Can you work these out from the model? Positions are in its coordinate system, mm. Give positions to 0.01 mm unless a question says otherwise; leave off trailing zeros. Order: outer loops, then holes, each group sorted by start corner. A loop starts at its lowest first (then second) coordinate and runs counter-clockwise, first axis right, second up. Notation, with made-up numbers: (27.25, -11.5) - (54.25, -11.5) arc R6 cw to (54.25, -5.5) - close; hole circle Ø4 at (-2.5, -18). An arc over 180 degrees is marked (long way). Return JSON: item names as keys, results as strings.
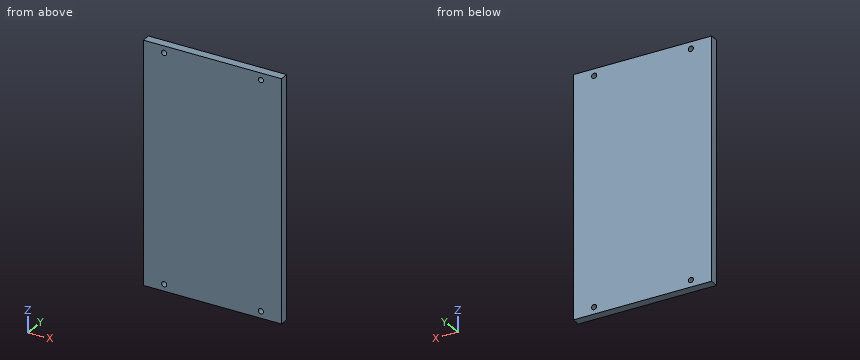
```python
from build123d import *

# Parameters (mm, degrees)
SKETCH1_W           = 80
SKETCH1_H           = 140
BOSS_EXTRUDE1_DEPTH = 5
SKETCH2_R           = 1.5
CUT_EXTRUDE1_DEPTH  = 162.322658049
SKETCH3_R           = 1.5
CUT_EXTRUDE2_DEPTH  = 162.322658049


with BuildPart() as part:
    # Sketch1 → Boss-Extrude1 (new body)
    with BuildSketch(Plane(origin=(0, 0, 0), x_dir=(1, 0, 0), z_dir=(0, 1, 0))):
        with Locations((-40, 70)):
            Rectangle(SKETCH1_W, SKETCH1_H)
    extrude(amount=BOSS_EXTRUDE1_DEPTH)

    # Sketch2 → Cut-Extrude1 (cut, through all)
    with BuildSketch(Plane(origin=(0, 5, 0), x_dir=(1, 0, 0), z_dir=(0, 1, 0))):
        with Locations(Location((-68, 136, 0), (0, 0, 270))):
            Circle(SKETCH2_R)
    cut_extrude1 = extrude(amount=-CUT_EXTRUDE1_DEPTH, mode=Mode.SUBTRACT)

    # Sketch3 → Cut-Extrude2 (cut, through all)
    with BuildSketch(Plane(origin=(0, 5, 0), x_dir=(1, 0, 0), z_dir=(0, 1, 0))):
        with Locations(Location((-12, 136, 0), (0, 0, 270))):
            Circle(SKETCH3_R)
    cut_extrude2 = extrude(amount=-CUT_EXTRUDE2_DEPTH, mode=Mode.SUBTRACT)

    # Mirror1: Cut-Extrude1, Cut-Extrude2 across plane
    add(cut_extrude1.mirror(Plane.XY.offset(-70)), mode=Mode.SUBTRACT)
    add(cut_extrude2.mirror(Plane.XY.offset(-70)), mode=Mode.SUBTRACT)


solid = part.part
```
1. If I drill on L1, parallel to Z at x = -68, y = 3.25; L2, parallel to X at y = 1.4, z = -4, over which ranges is the centre line in solid material (lowest first)? Write a range as [from, to].
Checks:
{"L1": "[-140, -137.5], [-134.5, -5.5], [-2.5, 0]", "L2": "[-80, -69.5], [-66.5, -13.5], [-10.5, 0]"}
2. Suppose I cut it at B-B (x = -68). List the corners of the cut face in (y, z) for me.
Checks:
{"outline": "(0, -140) - (5, -140) - (5, -137.5) - (0, -137.5) - close; (0, -134.5) - (5, -134.5) - (5, -5.5) - (0, -5.5) - close; (0, -2.5) - (5, -2.5) - (5, 0) - (0, 0) - close"}
3. Suppose I cut it at A-A (z = -136). List the corners of the cut face in (x, y) for me, plus the area to 3 significant figures.
Checks:
{"outline": "(-80, 0) - (-69.5, 0) - (-69.5, 5) - (-80, 5) - close; (-66.5, 0) - (-13.5, 0) - (-13.5, 5) - (-66.5, 5) - close; (-10.5, 0) - (0, 0) - (0, 5) - (-10.5, 5) - close", "area": "370 mm^2"}
